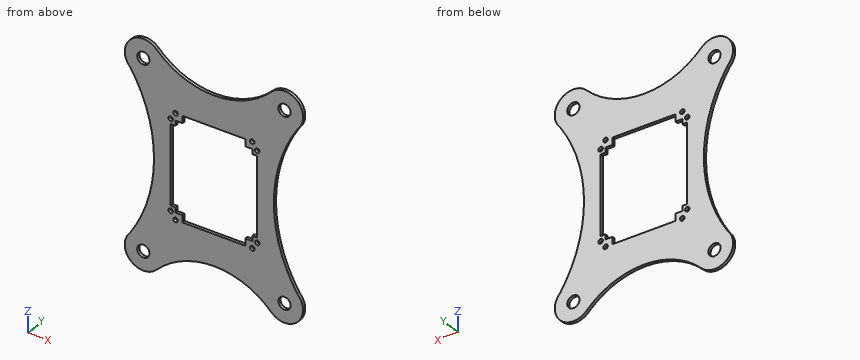
Autodesk Inventor part; units mm, degrees
ref_plane "YZ Plane" through (0, 0, 0) normal (1, 0, 0) x (0, 1, 0)
ref_plane "XZ Plane" through (0, 0, 0) normal (0, 1, 0) x (-1, 0, 0)
ref_plane "XY Plane" through (0, 0, 0) normal (0, 0, 1) x (1, 0, 0)
sketch "Sketch1" plane through (0, 0, 0) normal (0, 1, 0) x (-1, 0, 0)
  circle A0 centre (-28.625, 29.0323) radius 1.5
  circle A1 centre (-25.375, 33.6573) radius 1.5
  arc A2 (-37.9702, 69.5664) -> (0, 53.8386) centre (0, 107.5366) ccw
  arc A3 (-39.6019, 0) -> (-55.3297, 52.2069) centre (-134.1138, 0) ccw
  circle A4 centre (-46.65, 60.8866) radius 4.05
  arc A5 (-37.9702, 69.5664) -> (-55.3297, 52.2069) centre (-46.65, 60.8866) ccw
  arc A6 (-55.3297, -52.2069) -> (-39.6019, 0) centre (-134.1138, 0) ccw
  circle A7 centre (-28.625, -29.0323) radius 1.5
  circle A8 centre (-25.375, -33.6573) radius 1.5
  circle A9 centre (-46.65, -60.8866) radius 4.05
  arc A10 (-55.3297, -52.2069) -> (-37.9702, -69.5664) centre (-46.65, -60.8866) ccw
  arc A11 (0, -53.8386) -> (-37.9702, -69.5664) centre (0, -107.5366) ccw
  arc A12 (39.6019, 0) -> (55.3297, -52.2069) centre (134.1138, 0) ccw
  circle A13 centre (28.625, -29.0323) radius 1.5
  circle A14 centre (25.375, -33.6573) radius 1.5
  arc A15 (37.9702, -69.5664) -> (0, -53.8386) centre (0, -107.5366) ccw
  circle A16 centre (46.65, -60.8866) radius 4.05
  arc A17 (37.9702, -69.5664) -> (55.3297, -52.2069) centre (46.65, -60.8866) ccw
  circle A18 centre (28.625, 29.0323) radius 1.5
  circle A19 centre (25.375, 33.6573) radius 1.5
  arc A20 (0, 53.8386) -> (37.9702, 69.5664) centre (0, 107.5366) ccw
  arc A21 (55.3297, 52.2069) -> (39.6019, 0) centre (134.1138, 0) ccw
  circle A22 centre (46.65, 60.8866) radius 4.05
  arc A23 (55.3297, 52.2069) -> (37.9702, 69.5664) centre (46.65, 60.8866) ccw
  arc A24 (55.3297, 52.2069) -> (37.9702, 69.5664) centre (46.65, 60.8866) ccw
  arc A25 (-37.9702, 69.5664) -> (-55.3297, 52.2069) centre (-46.65, 60.8866) ccw
  arc A26 (-55.3297, -52.2069) -> (-37.9702, -69.5664) centre (-46.65, -60.8866) ccw
  circle A27 centre (-46.65, -60.8866) radius 4.05
  circle A28 centre (46.65, -60.8866) radius 4.05
  circle A29 centre (46.65, 60.8866) radius 4.05
  circle A30 centre (-46.65, 60.8866) radius 4.05
  circle A31 centre (-25.375, -33.6573) radius 1.5
  circle A32 centre (-28.625, -29.0323) radius 1.5
  circle A33 centre (25.375, -33.6573) radius 1.5
  circle A34 centre (28.625, -29.0323) radius 1.5
  circle A35 centre (28.625, 29.0323) radius 1.5
  circle A36 centre (25.375, 33.6573) radius 1.5
  circle A37 centre (-28.625, 29.0323) radius 1.5
  circle A38 centre (-25.375, 33.6573) radius 1.5
  arc A39 (-37.9702, 69.5664) -> (37.9702, 69.5664) centre (0, 107.5366) ccw
  arc A40 (55.3297, 52.2069) -> (55.3297, -52.2069) centre (134.1138, 0) ccw
  arc A41 (-55.3297, -52.2069) -> (-55.3297, 52.2069) centre (-134.1138, 0) ccw
  arc A42 (37.9702, -69.5664) -> (-37.9702, -69.5664) centre (0, -107.5366) ccw
  line L0 (28.625, -25.7823) -> (25.375, -25.7823)
  line L1 (25.375, 25.7823) -> (28.625, 25.7823)
  line L2 (28.625, 25.7823) -> (28.625, -25.7823)
  line L3 (-28.625, -25.7823) -> (-25.375, -25.7823)
  line L4 (-25.375, 25.7823) -> (-28.625, 25.7823)
  line L5 (-28.625, 25.7823) -> (-28.625, -25.7823)
  line L6 (20.75, -33.6573) -> (-20.75, -33.6573)
  line L7 (-20.75, -33.6573) -> (-20.75, -29.0323)
  line L8 (20.75, -29.0323) -> (20.75, -33.6573)
  line L9 (20.75, 33.6573) -> (-20.75, 33.6573)
  line L10 (-20.75, 33.6573) -> (-20.75, 29.0323)
  line L11 (20.75, 29.0323) -> (20.75, 33.6573)
  line L12 (25.375, 29.0323) -> (25.375, 25.7823)
  line L13 (25.375, -25.7823) -> (25.375, -29.0323)
  line L14 (25.375, -29.0323) -> (20.75, -29.0323)
  line L15 (-20.75, -29.0323) -> (-25.375, -29.0323)
  line L16 (-25.375, -29.0323) -> (-25.375, -25.7823)
  line L17 (-25.375, 25.7823) -> (-25.375, 29.0323)
  line L18 (-25.375, 29.0323) -> (-20.75, 29.0323)
  line L19 (20.75, 29.0323) -> (25.375, 29.0323)
  point P0 (-25.25, 18.3592)
  point P1 (-4.2075, 54.5249)
  point P2 (-4.2075, -54.5249)
  point P3 (25.25, 18.3592)
  point P4 (4.2075, -54.5249)
  point P5 (4.2075, 54.5249)
  dimension "d0" = 3.25
  dimension "d1" = 3.25
  dimension "d2" = 4.625
  dimension "d3" = 4.625
extrude "Extrusion1" add sketch "Sketch1" along normal blind 2
properties part number "atas4"
Check sheet for the modelled part. Datum: model origin and axes. Units: mm. Give positions to 0.01 mm unless a question says otherwise; leave off trailing zeros. Loops run counter-clockwise (first coordinate to the right, second up) from the corner with the lowest first, then second, coordinate; pieces in that order, holes last. Notation, with made-up numbers: M 32,9 L 81,9 A20 ccw 81,48 Z; hole C -15.5,28.25 d1. An arc over 180 degrees is marked long. Use a Markdown table: item, result. Add a question column.
Q1. Go/stop test with flat-tipped pins: pin 1 (1 mm diameter, centred on y = 0.5, z = -6, fed in from +X); pin 2 (1 mm diameter, centred on x = 23, y = 1, fed in from -Z); pin 3 (0.6 mm diameter, centred on x = -23, y = 1, fed in from +Z); pin 4 (2.5 mm diameter, centred on x = -25.38, z = -33.66, fed in from +Y). Record where each tip stops, or that it passes through.
Q2. Scan lines: line 1 along X through (y, z) = (1.5, -2) (3 decimals); line 2 along X through (y, z) = (1.8, 61.5); line 3 along Z through (x, y) = (46.65, 1.6). Record each from-to range of solid material in increasing order. Write a range as [from, to].
Q3. Sectioned sample at B-B, the plane x = -7. Record the cut outline in (y, z).
Q4. Sectioned sample at D-D, the plane y = 0.6. Give the number of separate pieces and of enclosed holes in the cut face, then the cut area to 3 significant figures.
Q5. Sectioned sample at A-A, the plane x = -46.65. Record the cut outline in (y, z).
Q6. Sectioned sample at C-C, the plane x = 19. Record the cut outline in (y, z).
Verdict:
| question | item | result |
|---|---|---|
| 1 | pin 1 | x = 39.83 |
| 1 | pin 2 | z = -59.25 |
| 1 | pin 3 | z = 59.16 |
| 1 | pin 4 | through |
| 2 | line 1 | [-39.623, -28.625], [28.625, 39.623] |
| 2 | line 2 | [-58.91, -50.65], [-42.65, -27.64], [27.64, 42.65], [50.65, 58.91] |
| 2 | line 3 | [-73.16, -64.94], [-56.84, -35.81], [35.81, 56.84], [64.94, 73.16] |
| 3 | outline | M 0,-54.3 L 2,-54.3 L 2,-33.66 L 0,-33.66 Z; M 0,33.66 L 2,33.66 L 2,54.3 L 0,54.3 Z |
| 4 | separate pieces | 1 |
| 4 | enclosed holes | 13 |
| 4 | area | 7,940 mm^2 |
| 5 | outline | M 0,-73.16 L 2,-73.16 L 2,-64.94 L 0,-64.94 Z; M 0,-56.84 L 2,-56.84 L 2,-35.81 L 0,-35.81 Z; M 0,35.81 L 2,35.81 L 2,56.84 L 0,56.84 Z; M 0,64.94 L 2,64.94 L 2,73.16 L 0,73.16 Z |
| 6 | outline | M 0,-57.31 L 2,-57.31 L 2,-33.66 L 0,-33.66 Z; M 0,33.66 L 2,33.66 L 2,57.31 L 0,57.31 Z |
